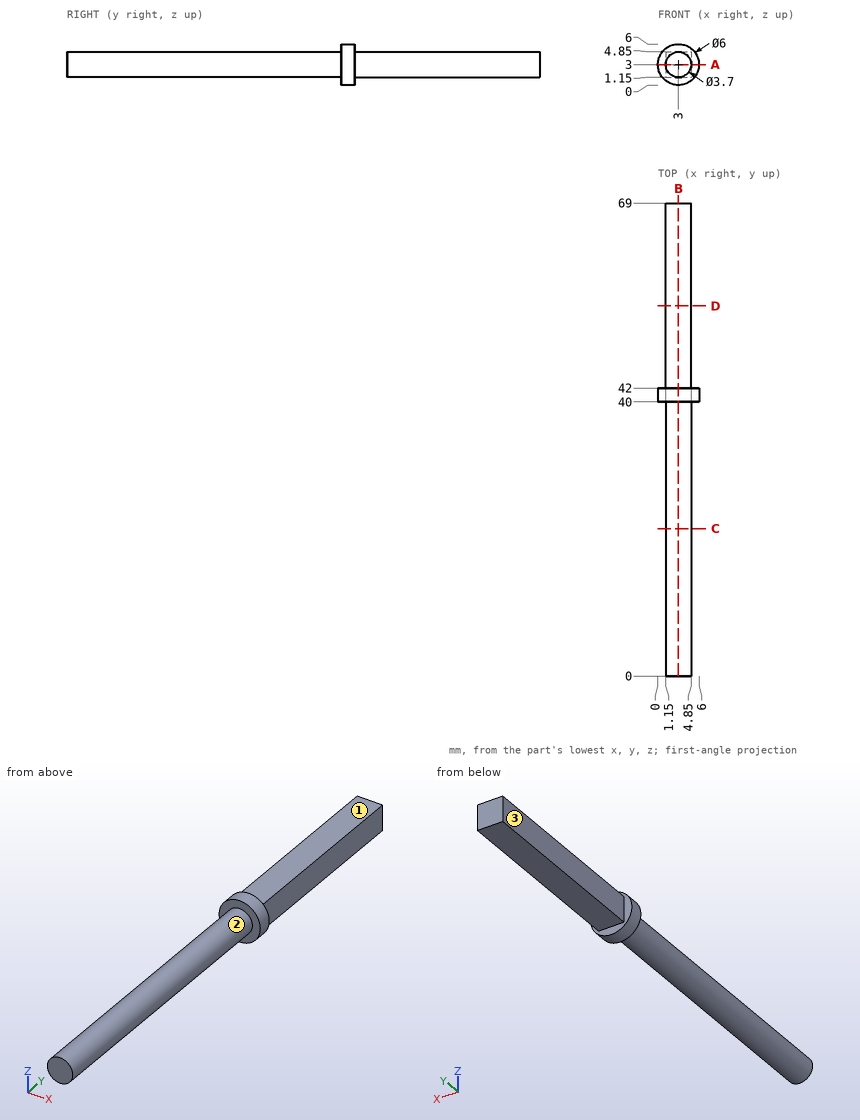
Can you work these out from the drawing? Everything is in mm from the part's minimum corner. A direction names the side the tool comes from. Give positions to 0.01 mm unless a question says otherwise; leave off trailing zeros. Loops run counter-clockwise (first coordinate to the right, second up) from the corner with the lowest first, then second, coordinate; pieces in that order, holes last. Notation, with made-up numbers: M 55,-38.5 L 89,-38.5 A29 cw 89,-13.5 Z; hole C 10,50 d5. An arc over 180 degrees is marked long. Use CSV: the item, a comma, the result in double quotes. Start each with the question number.
1. If I drill on L1, parallel to Z at x = 2.3, y = 51; L2, parallel to Y at x = 2.65, z = 0.5, over which ranges is the centre line in solid material (lowest first)?
2. For P1, Ø3, axis at y = 14, z = 3.5, coming from the -X side; P2, Ø1.8, axis at y = 58, z = 2, coming from the -X side; P3, Ø1.8, axis at x = 3, y = 49, coming from the +Z side, each with a flat end and sliding along its axis, tell me the tip position at first contact or that it passes through.
3. Imagine slicing it at B-B, the plane x = 3. Write out the boundary of the cut face in (y, z), plus the area to 3 significant figures.
4. Imagine slicing it at C-C, the plane y = 21.5. Write out the boundary of the cut face in (x, z), plus the area to 3 significant figures.
5. Imagine slicing it at A-A, the plane z = 3. Write out the boundary of the cut face in (x, y), plus the area to 3 significant figures.
6. On a 3-axis mill with a long thin cutter (end or side, diameter ignored), from which of +Z, -Z, +X, -X, +Y, -Y can I reach the whole of each face in a straight line? I mean the marked faces 1, 2 and 3. Say none if no direction works.
7. Imagine slicing it at D-D, the plane y = 54. Write out the boundary of the cut face in (x, z).
Response values:
1,L1,"1.15 to 4.85"
1,L2,"40 to 42"
2,P1,"x = 1.15"
2,P2,"x = 1.15"
2,P3,"z = 4.85"
3,outline,"M 0,1.15 L 40,1.15 L 40,0 L 42,0 L 42,1.15 L 69,1.15 L 69,4.85 L 42,4.85 L 42,6 L 40,6 L 40,4.85 L 0,4.85 Z"
3,area,"260 mm^2"
4,outline,"C 3,3 d3.7"
4,area,"10.8 mm^2"
5,outline,"M 0,40 L 1.15,40 L 1.15,0 L 4.85,0 L 4.85,40 L 6,40 L 6,42 L 4.85,42 L 4.85,69 L 1.15,69 L 1.15,42 L 0,42 Z"
5,area,"260 mm^2"
6,face 1,"+Z, +X, -X, +Y"
6,face 2,"-Y"
6,face 3,"+Z, -Z, -X, +Y"
7,outline,"M 1.15,1.15 L 4.85,1.15 L 4.85,4.85 L 1.15,4.85 Z"
